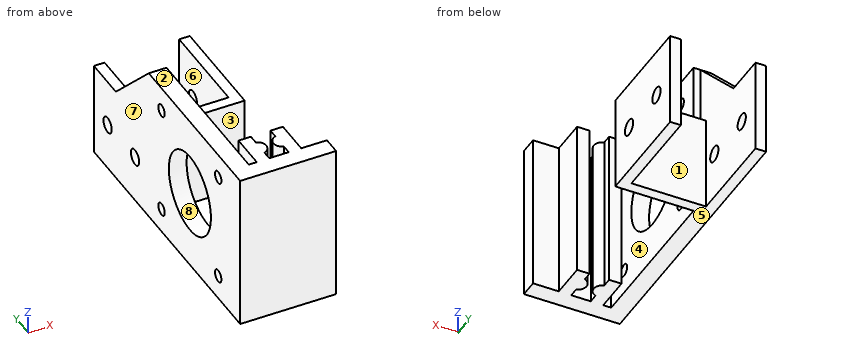
```python
from build123d import *

# Parameters (mm, degrees)
SKETCH1_W            = 27
SKETCH1_H            = 27
BOSS_EXTRUDE1_DEPTH  = 30
SKETCH2_W            = 21
SKETCH2_H            = 27
CUT_EXTRUDE1_DEPTH   = 30
SKETCH3_R            = 2.25
CUT_EXTRUDE2_DEPTH   = 30
SKETCH5_W            = 5
SKETCH5_H            = 45
BOSS_EXTRUDE2_DEPTH  = 45
SKETCH6_R            = 1.75
SKETCH6_R_2          = 11.5
CUT_EXTRUDE3_DEPTH   = 10
SKETCH8_W            = 45
SKETCH8_H            = 5
BOSS_EXTRUDE4_DEPTH  = 5
SKETCH9_W            = 45
SKETCH9_H            = 5
BOSS_EXTRUDE5_DEPTH  = 22
BOSS_EXTRUDE6_DEPTH  = 45
BOSS_EXTRUDE10_START = -3
BOSS_EXTRUDE10_DEPTH = 3


with BuildPart() as part:
    # Sketch1 → Boss-Extrude1 (new body)
    with BuildSketch(Plane(origin=(0, 0, 0), x_dir=(1, 0, 0), z_dir=(0, 1, 0))):
        Rectangle(SKETCH1_W, SKETCH1_H)
    extrude(amount=BOSS_EXTRUDE1_DEPTH)

    # Sketch2 → Cut-Extrude1 (cut)
    with BuildSketch(Plane(origin=(0, 0, -13.5), x_dir=(-1, 0, 0), z_dir=(0, 0, -1))):
        with Locations((0, 16.5)):
            Rectangle(SKETCH2_W, SKETCH2_H)
    extrude(amount=-CUT_EXTRUDE1_DEPTH, mode=Mode.SUBTRACT)

    # Sketch3 → Cut-Extrude2 (cut)
    with BuildSketch(Plane.ZY.offset(13.5)):
        with Locations((0, 7.5)):
            Circle(SKETCH3_R)
        with Locations((0, 22.5)):
            Circle(SKETCH3_R)
    extrude(amount=-CUT_EXTRUDE2_DEPTH, mode=Mode.SUBTRACT)

    # Sketch5 → Boss-Extrude2 (add)
    with BuildSketch(Plane.XZ):
        with Locations((-11, 9)):
            Rectangle(SKETCH5_W, SKETCH5_H)
    extrude(amount=BOSS_EXTRUDE2_DEPTH)

    # Sketch6 → Cut-Extrude3 (cut)
    with BuildSketch(Plane(origin=(-8.5, 0, 0), x_dir=(0, 0, -1), z_dir=(1, 0, 0))):
        with Locations((-24.5, -38)):
            Circle(SKETCH6_R)
        with Locations((-24.5, -7)):
            Circle(SKETCH6_R)
        with Locations((6.5, -7)):
            Circle(SKETCH6_R)
        with Locations((6.5, -38)):
            Circle(SKETCH6_R)
        with Locations((-9, -22.5)):
            Circle(SKETCH6_R_2)
    extrude(amount=-CUT_EXTRUDE3_DEPTH, mode=Mode.SUBTRACT)

    # Sketch8 → Boss-Extrude4 (add)
    with BuildSketch(Plane(origin=(-8.5, 0, 0), x_dir=(0, 0, -1), z_dir=(1, 0, 0))):
        with Locations((-9, -47.5)):
            Rectangle(SKETCH8_W, SKETCH8_H)
    extrude(amount=-BOSS_EXTRUDE4_DEPTH)

    # Sketch9 → Boss-Extrude5 (add)
    with BuildSketch(Plane(origin=(-8.5, 0, 0), x_dir=(0, 0, -1), z_dir=(1, 0, 0))):
        with Locations((-9, -47.5)):
            Rectangle(SKETCH9_W, SKETCH9_H)
    extrude(amount=BOSS_EXTRUDE5_DEPTH)

    # Sketch10 → Boss-Extrude6 (add)
    with BuildSketch(Plane.XY.offset(31.5)):
        with BuildLine():
            Line((-6.25, -35), (-6.25, -45))
            Line((-6.25, -45), (-2.75, -45))
            Line((-2.75, -45), (-2.75, -42.384848004))
            ThreePointArc((-2.75, -42.384848004), (-6, -40), (-2.75, -37.615151996))
            Line((-2.75, -37.615151996), (-2.75, -35))
            Line((-2.75, -35), (-6.25, -35))
        make_face()
        with BuildLine():
            ThreePointArc((-2.75, -37.615151996), (-6, -40), (-2.75, -42.384848004))
            Line((-2.75, -42.384848004), (-2.75, -37.615151996))
        make_face()
        with BuildLine():
            Line((-2.75, -37.615151996), (-2.75, -42.384848004))
            ThreePointArc((-2.75, -42.384848004), (-1.484435563, -41.479019946), (-1, -40))
            ThreePointArc((-1, -40), (-1.484435563, -38.520980054), (-2.75, -37.615151996))
        make_face()
        with BuildLine():
            ThreePointArc((2.75, -37.615151996), (1, -40), (2.75, -42.384848004))
            Line((2.75, -42.384848004), (2.75, -37.615151996))
        make_face()
        with BuildLine():
            Line((2.75, -37.615151996), (2.75, -42.384848004))
            ThreePointArc((2.75, -42.384848004), (4.979019946, -42.015564437), (6, -40))
            ThreePointArc((6, -40), (4.979019946, -37.984435563), (2.75, -37.615151996))
        make_face()
        with BuildLine():
            Line((2.75, -42.384848004), (2.75, -45))
            Line((2.75, -45), (6.25, -45))
            Line((6.25, -45), (6.25, -35))
            Line((6.25, -35), (2.75, -35))
            Line((2.75, -35), (2.75, -37.615151996))
            ThreePointArc((2.75, -37.615151996), (4.979019946, -37.984435563), (6, -40))
            ThreePointArc((6, -40), (4.979019946, -42.015564437), (2.75, -42.384848004))
        make_face()
    extrude(amount=-BOSS_EXTRUDE6_DEPTH)

    # Sketch15 → Boss-Extrude10 (add)
    with BuildSketch(Plane.ZY.offset(13.5).offset(BOSS_EXTRUDE10_START)):
        Polygon((31.5, 0), (13.5, 18), (13.5, 0), align=None)
    extrude(amount=BOSS_EXTRUDE10_DEPTH)


solid = part.part
```
Model file for the job. Use its own axes, mm. Face numbers are marked on the shaded views. A direction names the side the tool comes from. Round coordinates to 2 decimals unless told otherwise and drop trailing zeros. Write each loop counter-clockwise with the first axis right and the second up, starting at its lowest first coordinate (ties: lowest second). Pieces come first, ordered by that corner, then holes. Notation, with made-up numbers: (2.25, 15) -> (53.25, 15) arc R17 cw to (53.25, 37) -> close; hole circle Ø10 at (-26.75, 83). An arc over 180 degrees is marked (long way). Answer as CSV lines item,"result".
1. Pin check, flat tips, straight feed: pin 1 Ø10 at (x, y) = (8, 21) entering from +Z; pin 2 Ø0.6 at (x, z) = (-9, 22) entering from +Y; pin 3 Ø3 at (y, z) = (-38, 24.5) entering from +X; pin 4 Ø5 at (y, z) = (22.5, 0) entering from -X. Stop position of each tip, or through.
Resolved:
pin 1,"z = 13.5"
pin 2,"y = 0"
pin 3,"x = 6.25"
pin 4,"x = -13.5"
2. Tool access for the marked faces 1, 2, 3, 4 and 5: list every direction of +Z, -Z, +X, -X, +Y, -Y with a clear straight run to the whole face (end or side of a thin tool).
Resolved:
face 1,"+Z, -Z, +Y"
face 2,"+Z, +X, -X, +Y, -Y"
face 3,"+Z, -Z, +X"
face 4,"+Z, -Z"
face 5,"-Z, +X, -X, +Y, -Y"
3. Slice it at C-C, the plane y = 7.5. List the corners of the cut face in (x, z), plus the area to 4 significant figures.
Resolved:
outline,"(-13.5, -13.5) -> (-10.5, -13.5) -> (-10.5, -2.25) -> (-13.5, -2.25) -> close; (-13.5, 2.25) -> (-10.5, 2.25) -> (-10.5, 24) -> (-13.5, 24) -> close; (10.5, -13.5) -> (13.5, -13.5) -> (13.5, -2.25) -> (10.5, -2.25) -> close; (10.5, 2.25) -> (13.5, 2.25) -> (13.5, 13.5) -> (10.5, 13.5) -> close"
area,"166.5 mm²"
4. Slice it at A-A, the plane y = -7. List the corners of the cut face in (x, z), plus the area to 3 significant figures.
Resolved:
outline,"(-13.5, -13.5) -> (-8.5, -13.5) -> (-8.5, -8.25) -> (-13.5, -8.25) -> close; (-13.5, -4.75) -> (-8.5, -4.75) -> (-8.5, 22.75) -> (-13.5, 22.75) -> close; (-13.5, 26.25) -> (-8.5, 26.25) -> (-8.5, 31.5) -> (-13.5, 31.5) -> close"
area,"190 mm²"
5. Drill centre lines: line 1 (X direction, y = -43.5, z = 1.5); line 2 (Y direction, x = -9.55, z = 24.5); line 3 (X direction, y = 16, z = 9). Where is each one in solid material? Low to high.
Resolved:
line 1,"-13.5 to -8.5, -6.25 to -2.75, 2.75 to 6.25"
line 2,"-50 to -39.75, -36.25 to -8.75, -5.25 to 0"
line 3,"-13.5 to -10.5, 10.5 to 13.5"
6. Slice it at D-D, the plane y = -22.5. List the corners of the cut face in (x, z), plus the area to 3 significant figures.
Resolved:
outline,"(-13.5, -13.5) -> (-8.5, -13.5) -> (-8.5, -2.5) -> (-13.5, -2.5) -> close; (-13.5, 20.5) -> (-8.5, 20.5) -> (-8.5, 31.5) -> (-13.5, 31.5) -> close"
area,"110 mm²"
7. Slice it at B-B, the plane x = 0. List the corners of the cut face in (y, z), plus the area to 3 significant figures.
Resolved:
outline,"(-50, -13.5) -> (-45, -13.5) -> (-45, 31.5) -> (-50, 31.5) -> close; (0, -13.5) -> (3, -13.5) -> (3, 13.5) -> (0, 13.5) -> close"
area,"306 mm²"
8. Mould opens along X. For the marked faces 6, 7 and 8 say: +X half, -X half, draft (parallel to the pull), parting line (faces both ways), or undercut.
Resolved:
face 6,"undercut"
face 7,"-X half"
face 8,"draft"
